```python
from build123d import *

# Parameters (mm, degrees)
F0_W     = 130
F0_H     = 75
F1_DEPTH = 75
F3_DEPTH = 90
F4_W     = 70
F4_H     = 45
F5_DEPTH = 25


with BuildPart() as f1:
    # F0 (on Top) → F1 (new body)
    with BuildSketch(Plane.XY):
        with Locations((65, 37.5)):
            Rectangle(F0_W, F0_H)
    extrude(amount=F1_DEPTH)

    # F2 (on face) → F3 (cut)
    with BuildSketch(Plane.XY.offset(75)):
        Polygon((0, 0), (105, 0), (105, 30), (80, 30), (80, 45), (55, 45), (55, 30), (0, 30), align=None)
    extrude(amount=-F3_DEPTH, mode=Mode.SUBTRACT)

    # F4 (on face) → F5 (cut)
    with BuildSketch(Plane.XY.offset(75)):
        with Locations((57.5, 52.5)):
            Rectangle(F4_W, F4_H)
    extrude(amount=-F5_DEPTH, mode=Mode.SUBTRACT)


solid = f1.part
```
Design review of the part built by this model. Coordinates are the model's own, in mm. A direction names the side the tool comes from. Coordinates: 2 decimals unless noted, no trailing zeros. Order: outer loops, then holes, each group sorted by start corner. A loop starts at its lowest first (then second) coordinate and runs counter-clockwise, first axis right, second up.
1) Take a section at D-D, the plane y = 70. Give the boundary of the cut face in (x, z).
2) For faces 4 (the flat face through (105, 15, 38)), 5 (the flat face through (22.5, 52, 63)), 6 (the flat face through (55, 38, 25)), list the 3-axis set-ups (+Z, -Z, +X, -X, +Y, -Y) from which the entire face can be reached by the end or side of a thin tool; tool diameter is ignored.
3) Take a section at C-C, the plane z = 19.5. Give the boundary of the cut face in (x, y), and give its area (4 significant figures).
4) Take a section at A-A, the plane z = 58. Give the boundary of the cut face in (x, y).
5) Mouldability with a two-part tool opening along X and no side actions: class faces 1 (the flat face through (0, 52, 37)), 2 (the flat face through (68, 45, 25)), 3 (the flat face through (28, 30, 30)) as +X half, -X half, draft (parallel to the pull), parting line (faces both ways), or undercut.
6) Wall thickness on line 1 along X through (y, z) = (38, 23.5); line 2 along X through (y, z) = (48.5, 56.5); line 3 along Z through (x, y) = (45, 44): over which ranges is each line inside the solid? List them lowest first.
7) Take a section at B-B, the plane y = 41.5. Give the boundary of the cut face in (x, z), and give its area (3 significant figures).
8) Clearance check with flat-ended pins moving along their axes: pin 1 (12.5 mm diameter, centred on x = 65, z = 28.5, fed in from -Y); pin 2 (6 mm diameter, centred on x = 54.5, z = 19, fed in from -Y); pin 3 (1 mm diameter, centred on y = 24.5, z = 54, fed in from -X). State where each tip first meets the part, or that it passes through.
Returned:
1. outline: (0, 0) - (130, 0) - (130, 75) - (92.5, 75) - (92.5, 50) - (22.5, 50) - (22.5, 75) - (0, 75) - close
2. face 4: +Z, -Z, -X, -Y
2. face 5: +Z, +Y, -Y
2. face 6: +Z, -Z, -Y
3. outline: (0, 30) - (55, 30) - (55, 45) - (80, 45) - (80, 30) - (105, 30) - (105, 0) - (130, 0) - (130, 75) - (0, 75) - close
3. area: 6,225 mm2
4. outline: (0, 30) - (22.5, 30) - (22.5, 75) - (0, 75) - close; (92.5, 30) - (105, 30) - (105, 0) - (130, 0) - (130, 75) - (92.5, 75) - close
5. face 1: -X half
5. face 2: undercut
5. face 3: draft
6. line 1: x = 0 to 55, 80 to 130
6. line 2: x = 0 to 22.5, 92.5 to 130
6. line 3: z = 0 to 50
7. outline: (0, 0) - (55, 0) - (55, 50) - (22.5, 50) - (22.5, 75) - (0, 75) - close; (80, 0) - (130, 0) - (130, 75) - (92.5, 75) - (92.5, 50) - (80, 50) - close
7. area: 6,750 mm2
8. pin 1: stops at y = 45
8. pin 2: stops at y = 30
8. pin 3: stops at x = 105
